Check sheet for the drawn part. Datum: minimum x, y, z corner. Units: mm. A direction names the side the tool comes from. Coordinates: 2 decimals unless noted, no trailing zeros. Loops run counter-clockwise (first coordinate to the right, second up) from the corner with the lowest first, then second, coordinate; pieces in that order, holes last.
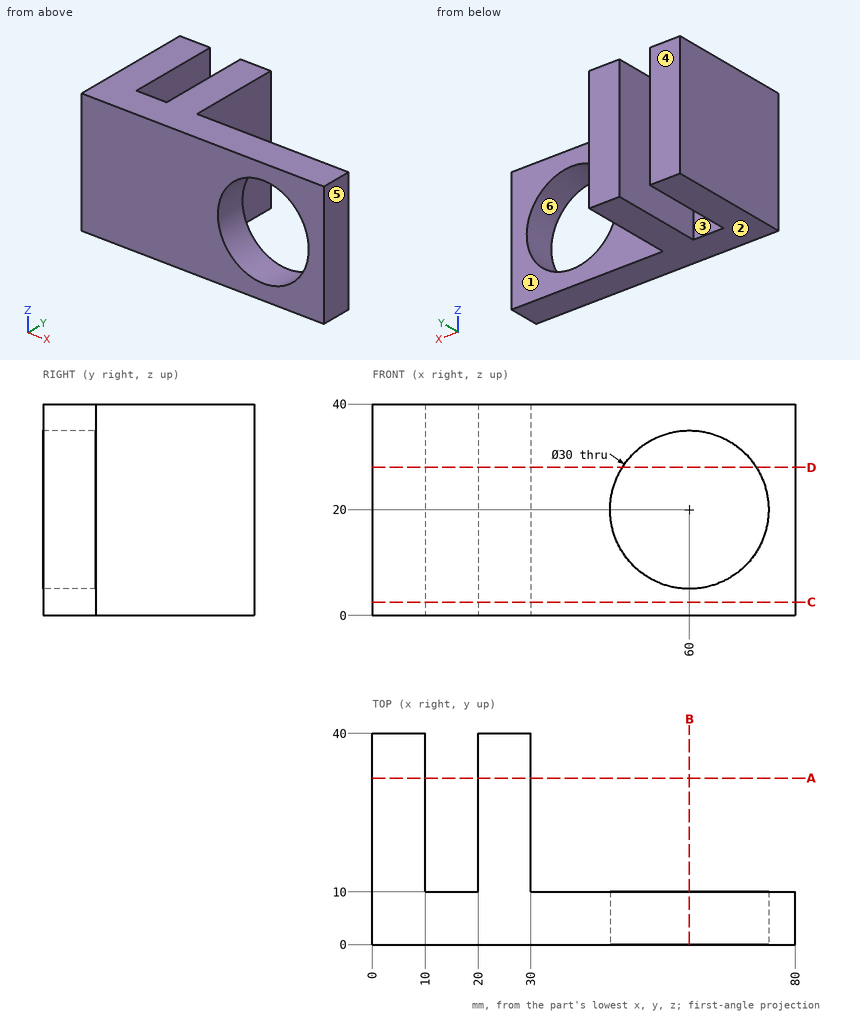
1) Section check B-B on x = 60. Enter the section's corners in (y, z), plus the area to 3 significant figures.
Answer sheet:
outline: (0, 0) - (10, 0) - (10, 5) - (0, 5) - close; (0, 35) - (10, 35) - (10, 40) - (0, 40) - close
area: 100 mm2
2) Depth check by flat-ended pin: pin 1 (18 mm diameter, centred on x = 60, z = 20, fed in from +Y); pin 2 (6 mm diameter, centred on x = 61.5, z = 36, fed in from +Y). Enter the tip coordinate at first touch or a pass-through.
Answer sheet:
pin 1: passes through
pin 2: stops at y = 10
3) Section check D-D on z = 28. Enter the section's corners in (x, y).
Answer sheet:
outline: (0, 0) - (47.31, 0) - (47.31, 10) - (30, 10) - (30, 40) - (20, 40) - (20, 10) - (10, 10) - (10, 40) - (0, 40) - close; (72.69, 0) - (80, 0) - (80, 10) - (72.69, 10) - close
4) Set-up check for the marked faces 1, 2 and 3: record each of +Z, -Z, +X, -X, +Y, -Y from which the full face is reachable in a straight line by a thin tool's end or side.
Answer sheet:
face 1: +Z, -Z, +X, +Y
face 2: -Z, +X, -X, +Y, -Y
face 3: +Z, -Z, +Y
5) Scan lines: line 1 (X direction, y = 34, z = 34); line 2 (X direction, y = 2.25, z = 20); line 3 (Y direction, x = 75, z = 3). Record each from-to range of solid material in increasing order.
Answer sheet:
line 1: x = 0 to 10, 20 to 30
line 2: x = 0 to 45, 75 to 80
line 3: y = 0 to 10
6) Section check A-A on y = 31.5. Enter the section's corners in (x, z).
Answer sheet:
outline: (0, 0) - (10, 0) - (10, 40) - (0, 40) - close; (20, 0) - (30, 0) - (30, 40) - (20, 40) - close
7) Mould release check, pull along X, two halves, no side actions. Record for the marked faces 4, 5 and 6: +X half, -X half, draft (parallel to the pull), parting line (faces both ways), or undercut.
Answer sheet:
face 4: draft
face 5: +X half
face 6: undercut
8) Section check C-C on z = 2.5. Enter the section's corners in (x, y), plus the area to 3 significant figures.
Answer sheet:
outline: (0, 0) - (80, 0) - (80, 10) - (30, 10) - (30, 40) - (20, 40) - (20, 10) - (10, 10) - (10, 40) - (0, 40) - close
area: 1,400 mm2
